from build123d import *

# Parameters (mm, degrees)
SKETCH_1_W             = 1000
SKETCH_1_H             = 100
EXTRUDE_1_DEPTH        = 20
SKETCH_2_W             = 1000
SKETCH_2_H             = 30
EXTRUDE_2_DEPTH        = 242
EXTRUDE_START          = -30
EXTRUDE_3_DEPTH        = 10
PATTERN_LINEAR_1_COUNT = 3
PATTERN_LINEAR_1_PITCH = 380
CUT_EXTRUDE_1_DEPTH    = 574.274803214


with BuildPart() as part:
    # Sketch 1 → Extrude 1 (new body)
    with BuildSketch(Plane.XY):
        Rectangle(SKETCH_1_W, SKETCH_1_H)
    extrude(amount=EXTRUDE_1_DEPTH)



with BuildPart() as body_2:
    # Sketch 2 → Extrude 2 (new body)
    with BuildSketch(Plane.XY.offset(20)):
        with Locations((0, 35)):
            Rectangle(SKETCH_2_W, SKETCH_2_H)
    extrude(amount=EXTRUDE_2_DEPTH)


with BuildPart() as part_1:
    add(part.part)

    add(body_2.part)  # Extrude 3 merges body 2
    # Sketch 3 → Extrude 3 (add)
    with BuildSketch(Plane.ZY.offset(500).offset(EXTRUDE_START)):
        Polygon((262, 20), (20, 20), (20, -50), (40, -50), (262, 0), align=None)
    extrude_3 = extrude(amount=-EXTRUDE_3_DEPTH)

    # Pattern Linear 1: Extrude 3 ×3
    with Locations(*[(i * PATTERN_LINEAR_1_PITCH, 0, 0) for i in range(1, PATTERN_LINEAR_1_COUNT)]):
        add(extrude_3)

    # Sketch 5 → Cut-Extrude 1 (cut, through all)
    with BuildSketch(Plane(origin=(0, 50, 0), x_dir=(1, 0, 0), z_dir=(0, 1, 0))):
        with BuildLine():
            Line((357.5, -256.999999998), (357.5, -337.435999102))
            ThreePointArc((357.5, -337.435999102), (340, -354.935999102), (322.5, -337.435999102))
            Line((322.5, -337.435999102), (322.5, -256.999999998))
            ThreePointArc((322.5, -256.999999998), (340, -239.499999998), (357.5, -256.999999998))
        make_face()
        with BuildLine():
            Line((-322.5, -257), (-322.5, -349.000883912))
            ThreePointArc((-322.5, -349.000883912), (-340, -366.500883912), (-357.5, -349.000883912))
            Line((-357.5, -349.000883912), (-357.5, -257))
            ThreePointArc((-357.5, -257), (-340, -239.5), (-322.5, -257))
        make_face()
    extrude(amount=-CUT_EXTRUDE_1_DEPTH, mode=Mode.SUBTRACT)


solid = part_1.part
Can you work these out from the model? Positions are in its coordinate system, mm. A direction names the side the tool comes from. Coordinates: 2 decimals unless noted, no trailing zeros. Order: outer loops, then holes, each group sorted by start corner. A loop starts at its lowest first (then second) coordinate and runs counter-clockwise, first axis right, second up. Notation, with made-up numbers: M 65,31 L 103,31 A29 ccw 103,60 Z; hole C 7,1.25 d10. An arc over 180 degrees is marked long. Write item = value, one per line.
(1) Suppose I cut it at A-A on y = -16. Please give me the cut outline in (x, z), plus the area to 3 significant figures.
Results are:
outline = M -500,0 L 500,0 L 500,20 L 300,20 L 300,190.96 L 290,190.96 L 290,20 L -80,20 L -80,190.96 L -90,190.96 L -90,20 L -460,20 L -460,190.96 L -470,190.96 L -470,20 L -500,20 Z
area = 25,100 mm2
(2) For pin 1 Ø4 at (x, y) = (-86.5, -34) entering from -Z; pin 2 Ø6 at (x, z) = (272.5, 199.5) entering from -Y; pin 3 Ø4 at (y, z) = (-1.5, 101) entering from -X, each with a flat end and sliding along its axis, tell me the tip position at first contact or that it passes through.
Results are:
pin_1 = 0
pin_2 = 20
pin_3 = -470
(3) Suppose I cut it at D-D on x = -340. Please give me the cut outline in (y, z), plus the area to 4 significant figures.
Results are:
outline = M -50,0 L 50,0 L 50,239.5 L 20,239.5 L 20,20 L -50,20 Z
area = 8,585 mm2
(4) Suppose I cut it at C-C on z = 150.5. Please give me the cut outline in (x, y).
Results are:
outline = M -500,20 L -470,20 L -470,-25.11 L -460,-25.11 L -460,20 L -90,20 L -90,-25.11 L -80,-25.11 L -80,20 L 290,20 L 290,-25.11 L 300,-25.11 L 300,20 L 500,20 L 500,50 L -500,50 Z
(5) I need wall thicknesses on line 1 along X through (y, z) = (-29, 87.5); line 2 along Z through (x, y) = (-60, -33.5); line 3 along Y through (x, z) = (327.5, 56). Which ranges of each line are inside material? Lowest first, please. Write a range as [from, to].
Results are:
line_1 = [-470, -460], [-90, -80], [290, 300]
line_2 = [0, 20]
line_3 = [20, 50]
(6) For faces 4 (the face through (-80, -7, 112)), 5 (the face through (-485, 20, 139)), 6 (the face through (339.615, 35.21, 239.504)), which set-ups out of +Z, -Z, +X, -X, +Y, -Y let a thin tool reach every point of the face, with its end or its side?
Results are:
face_4 = +Z, -Y
face_5 = +Z, -X, -Y
face_6 = +Z, +Y, -Y
(7) Suppose I cut it at B-B on x = -145. Please give me the cut outline in (y, z).
Results are:
outline = M -50,0 L 50,0 L 50,262 L 20,262 L 20,20 L -50,20 Z
(8) If we mould it in two halves opening along X, with no side actions, what happens to faces 1 (the face through (300, -7, 112)), 2 (the face through (290, -7, 112)), 3 (the face through (-85.07, -25.35, 149.45))? For each: pulls with the +X half, pulls with the -X half, needs draft (parallel to the pull), parting line crosses it, or undercut.
Results are:
face_1 = pulls with the +X half
face_2 = undercut
face_3 = needs draft
